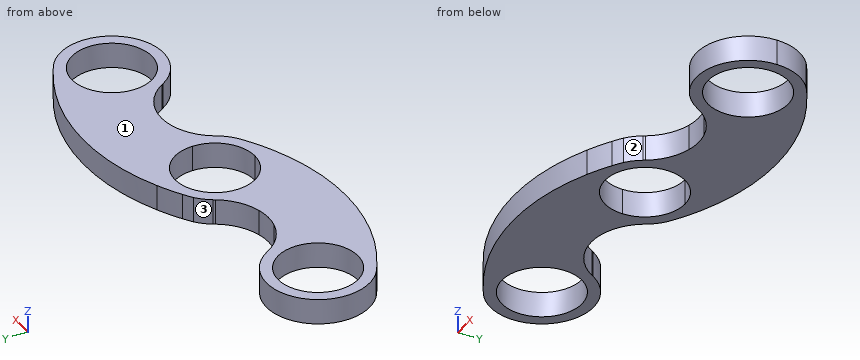
```python
from build123d import *

# Parameters (mm, degrees)
F0_R     = 11
F1_DEPTH = 7


with BuildPart() as f1:
    # F0 (on Top) → F1 (new body)
    with BuildSketch(Plane.XY):
        with BuildLine():
            Line((14.175, 0), (11, 0))
            ThreePointArc((11, 0), (7.7781745931, -7.7781745931), (0, -11))
            Line((0, -11), (0, -14.175))
            ThreePointArc((0, -14.175), (3.2814696071, -13.7899449679), (6.3846610647, -12.655699431))
            ThreePointArc((6.3846610647, -12.655699431), (7.6740188796, -11.8429761162), (8.9426071008, -10.9982))
            ThreePointArc((8.9426071008, -10.9982), (10.6919977036, -9.3065466262), (12.1262614453, -7.3406))
            ThreePointArc((12.1262614453, -7.3406), (12.2596266851, -7.1057126256), (12.3971479741, -6.8732341084))
            ThreePointArc((12.3971479741, -6.8732341084), (13.7233413849, -3.5497219939), (14.175, 0))
        make_face()
        with BuildLine():
            ThreePointArc((0, 11), (7.7781745931, 7.7781745931), (11, 0))
            Line((11, 0), (14.175, 0))
            ThreePointArc((14.175, 0), (10.0232386233, 10.0232386233), (0, 14.175))
            Line((0, 14.175), (0, 11))
        make_face()
        with BuildLine():
            ThreePointArc((-11, 0), (-7.7781745931, 7.7781745931), (0, 11))
            Line((0, 11), (0, 14.175))
            ThreePointArc((0, 14.175), (-3.2888623779, 13.7881836824), (-6.3982276645, 12.6488461036))
            ThreePointArc((-6.3982276645, 12.6488461036), (-7.6795852422, 11.8402648338), (-8.9403928885, 11))
            ThreePointArc((-8.9403928885, 11), (-10.6938487189, 9.304419626), (-12.1306573285, 7.3333333333))
            ThreePointArc((-12.1306573285, 7.3333333333), (-12.2610462299, 7.103700791), (-12.3954086387, 6.8763703856))
            ThreePointArc((-12.3954086387, 6.8763703856), (-13.7228922326, 3.5514579785), (-14.175, 0))
            Line((-14.175, 0), (-11, 0))
        make_face()
        with BuildLine():
            Line((0, -14.175), (0, -11))
            ThreePointArc((0, -11), (-7.7781745931, -7.7781745931), (-11, 0))
            Line((-11, 0), (-14.175, 0))
            ThreePointArc((-14.175, 0), (-10.0232386233, -10.0232386233), (0, -14.175))
        make_face()
        with BuildLine():
            ThreePointArc((0, 14.175), (10.0232386233, 10.0232386233), (14.175, 0))
            Line((14.175, 0), (21.6662, 0))
            ThreePointArc((21.6662, 0), (25.4, 0.4661082384), (29.1338, 0))
            Line((29.1338, 0), (36.625, 0))
            ThreePointArc((36.625, 0), (43.3747333645, 12.0746031153), (57.1958698966, 12.650038469))
            ThreePointArc((57.1958698966, 12.650038469), (29.0258725789, 21.5203456529), (0, 16.0678398574))
            Line((0, 16.0678398574), (0, 14.175))
        make_face()
        with BuildLine():
            Line((21.6662, 0), (14.175, 0))
            ThreePointArc((14.175, 0), (13.7233413849, -3.5497219939), (12.3971479741, -6.8732341084))
            ThreePointArc((12.3971479741, -6.8732341084), (16.353496972, -2.5220464261), (21.6662, 0))
        make_face()
        with BuildLine():
            ThreePointArc((-6.3982276645, 12.6488461036), (-3.2888623779, 13.7881836824), (0, 14.175))
            Line((0, 14.175), (0, 16.0678398574))
            ThreePointArc((0, 16.0678398574), (-3.2501607804, 14.453871086), (-6.3982276645, 12.6488461036))
        make_face()
        with BuildLine():
            Line((0, -16.0641572656), (0, -14.175))
            ThreePointArc((0, -14.175), (-10.0232386233, -10.0232386233), (-14.175, 0))
            Line((-14.175, 0), (-21.6559333333, 0))
            ThreePointArc((-21.6559333333, 0), (-25.4, -0.4688166689), (-29.1440666667, 0))
            Line((-29.1440666667, 0), (-36.625, 0))
            ThreePointArc((-36.625, 0), (-43.3693858125, -12.0713130104), (-57.1846610647, -12.655699431))
            ThreePointArc((-57.1846610647, -12.655699431), (-29.0187526069, -21.5141320936), (0, -16.0641572656))
        make_face()
        with BuildLine():
            ThreePointArc((6.3846610647, -12.655699431), (3.2814696071, -13.7899449679), (0, -14.175))
            Line((0, -14.175), (0, -16.0641572656))
            ThreePointArc((0, -16.0641572656), (3.2430752796, -14.4549824836), (6.3846610647, -12.655699431))
        make_face()
        with BuildLine():
            Line((-21.6559333333, 0), (-14.175, 0))
            ThreePointArc((-14.175, 0), (-13.7228922326, 3.5514579785), (-12.3954086387, 6.8763703856))
            ThreePointArc((-12.3954086387, 6.8763703856), (-16.3473482418, 2.5246764417), (-21.6559333333, 0))
        make_face()
        with BuildLine():
            Line((36.625, 0), (29.1338, 0))
            ThreePointArc((29.1338, 0), (34.446503028, -2.5220464261), (38.4028520259, -6.8732341084))
            ThreePointArc((38.4028520259, -6.8732341084), (37.0766586151, -3.5497219939), (36.625, 0))
        make_face()
        with BuildLine():
            ThreePointArc((59.7426071008, 10.9982), (58.47955068, 11.8400181351), (57.1958698966, 12.650038469))
            ThreePointArc((57.1958698966, 12.650038469), (43.3747333645, 12.0746031153), (36.625, 0))
            ThreePointArc((36.625, 0), (37.0766586151, -3.5497219939), (38.4028520259, -6.8732341084))
            ThreePointArc((38.4028520259, -6.8732341084), (38.5403733149, -7.1057126256), (38.6737385547, -7.3406))
            ThreePointArc((38.6737385547, -7.3406), (54.6105687904, -13.6532117281), (64.975, 0))
            ThreePointArc((64.975, 0), (63.6002359481, 6.0897113784), (59.7426071008, 10.9982))
        make_face()
        with BuildLine():
            ThreePointArc((61.8, 0), (50.8, -11), (39.8, 0))
            ThreePointArc((39.8, 0), (50.8, 11), (61.8, 0))
        make_face(mode=Mode.SUBTRACT)
        with BuildLine():
            ThreePointArc((-59.7426071008, -10.9982), (-58.4740188796, -11.8429761162), (-57.1846610647, -12.655699431))
            ThreePointArc((-57.1846610647, -12.655699431), (-43.3693858125, -12.0713130104), (-36.625, 0))
            ThreePointArc((-36.625, 0), (-37.0771077674, 3.5514579785), (-38.4045913613, 6.8763703856))
            ThreePointArc((-38.4045913613, 6.8763703856), (-38.5389537701, 7.103700791), (-38.6693426715, 7.3333333333))
            ThreePointArc((-38.6693426715, 7.3333333333), (-60.1033431975, 10.6947851941), (-59.7426071008, -10.9982))
        make_face()
        with Locations((-50.8, 0)):
            Circle(F0_R, mode=Mode.SUBTRACT)
        with BuildLine():
            Line((-36.625, 0), (-29.1440666667, 0))
            ThreePointArc((-29.1440666667, 0), (-34.4526517582, 2.5246764417), (-38.4045913613, 6.8763703856))
            ThreePointArc((-38.4045913613, 6.8763703856), (-37.0771077674, 3.5514579785), (-36.625, 0))
        make_face()
    extrude(amount=F1_DEPTH)


solid = f1.part
```
Work out the finished part from the listing and answer in its coordinate system (mm). Face numbers are marked on the shaded views. Give positions to 0.01 mm unless a question says otherwise; leave off trailing zeros. Loops run counter-clockwise (first coordinate to the right, second up) from the corner with the lowest first, then second, coordinate; pieces in that order, holes last. Notation, with made-up numbers: (42, 63) -> (79, 63) arc R23 ccw to (79, 78) -> close; hole circle Ø5 at (-9, -14). An arc over 180 degrees is marked (long way). One line per question, with ' | ' between items. Start each with the question number.
1) Straight lines are drawn through the part: L1, parallel to Y at x = 50.8, z = 3 (3 decimals); L2, parallel to X at y = -9.5, z = 2.5; L3, parallel to X at y = -4, z = 5.5. For each, find the intervals that lie inside material, in ascending order.
2) Section B-B, the plane z = 5.5 is taken. Determine the outline of the cut face in (x, y) (3 decimals), then the cut area to 3 significant figures.
3) Section C-C, the plane x = 50.8 is taken. Determine the outline of the cut face in (y, z) (3 decimals), then the cut area to 3 significant figures.
4) Each of these flat-tipped pins is pushed along its axis until it touches: pin 1 (1.5 mm diameter, centred on y = 0.5, z = 1.5, fed in from -X) (3 decimals); pin 2 (2 mm diameter, centred on y = -4, z = 2.5, fed in from -X); pin 3 (4 mm diameter, centred on x = -45.5, z = 4, fed in from +Y); pin 4 (1.5 mm diameter, centred on y = 10, z = 6, fed in from +X). Where does it stop, or does it pass through?
5) Determine the mould class of the marked faces 1, 2 and 3 for opening direction X: +X half, -X half, draft (parallel to the pull), parting line (faces both ways), or undercut.
6) Section A-A, the plane x = -50.8 is taken. Determine the outline of the cut face in (y, z) (3 decimals), then the cut area to 3 significant figures.
Resolved:
1) L1: -14.175 to -11, 11 to 16.068 | L2: -61.32 to -56.35, -45.25 to -5.55, 5.55 to 10.52, 40.28 to 45.25, 56.35 to 61.32 | L3: -64.4 to -61.05, -40.55 to -10.25, 10.25 to 14.64, 36.16 to 40.55, 61.05 to 64.4
2) outline: (-59.743, -10.998) arc R60.821 ccw to (8.943, -10.998) arc R14.175 ccw to (12.126, -7.341) arc R15.188 cw to (38.674, -7.341) arc R14.175 ccw (long way) to (59.743, 10.998) arc R60.79 ccw to (-8.94, 11) arc R14.175 ccw to (-12.131, 7.333) arc R15.185 cw to (-38.669, 7.333) arc R14.175 ccw (long way) to start; hole circle Ø22 at (-50.8, 0); hole circle Ø22 at (0, 0); hole circle Ø22 at (50.8, 0) | area: 2,210 mm2
3) outline: (-14.175, 0) -> (-11, 0) -> (-11, 7) -> (-14.175, 7) -> close; (11, 0) -> (16.068, 0) -> (16.068, 7) -> (11, 7) -> close | area: 57.7 mm2
4) pin 1: x = -64.975 | pin 2: x = -64.65 | pin 3: y = 13.79 | pin 4: x = 61.54
5) face 1: draft | face 2: undercut | face 3: undercut
6) outline: (-16.064, 0) -> (-11, 0) -> (-11, 7) -> (-16.064, 7) -> close; (11, 0) -> (14.175, 0) -> (14.175, 7) -> (11, 7) -> close | area: 57.7 mm2
